Read the model definition and answer for the solid it produces. Units are mm, in the model's axes. A direction names the side the tool comes from. Coordinates: 2 decimals unless noted, no trailing zeros. Order: outer loops, then holes, each group sorted by start corner. A loop starts at its lowest first (then second) coordinate and runs counter-clockwise, first axis right, second up. Notation, with made-up numbers: (34.25, 31) -> (72.25, 31) arc R11 ccw to (72.25, 46) -> close; hole circle Ø8 at (8, 64). An arc over 180 degrees is marked (long way). Answer in a Markdown table with one row per item.
from build123d import *

# Parameters (mm, degrees)
SKETCH_1_R          = 7
EXTRUDE_1_DEPTH     = 2
SKETCH_2_R          = 5
EXTRUDE_2_DEPTH     = 5
SKETCH_3_R          = 2.5
CUT_EXTRUDE_1_DEPTH = 5
FILLET_1_R          = 1


with BuildPart() as part:
    # 草图1 → 凸台-拉伸1 (new body)
    with BuildSketch(Plane(origin=(0, 0, 0), x_dir=(1, 0, 0), z_dir=(0, 1, 0))):
        Circle(SKETCH_1_R)
    extrude(amount=EXTRUDE_1_DEPTH)

    # 草图2 → 凸台-拉伸2 (add)
    with BuildSketch(Plane(origin=(0, 2, 0), x_dir=(1, 0, 0), z_dir=(0, 1, 0))):
        Circle(SKETCH_2_R)
    extrude(amount=EXTRUDE_2_DEPTH)

    # 草图3 → 切除-拉伸1 (cut)
    with BuildSketch(Plane.XZ):
        Circle(SKETCH_3_R)
    extrude(amount=-CUT_EXTRUDE_1_DEPTH, mode=Mode.SUBTRACT)

    # 圆角1
    fillet_1_edges = [part.edges().sort_by_distance(p)[0] for p in [
        (-5, 7, 0),
    ]]
    fillet(fillet_1_edges, radius=FILLET_1_R)


solid = part.part
Q1. For faces 1 (the face through (-1.08, 3.97, 4.88)), 2 (the face through (-0.54, 2.46, -2.44)), 3 (the face through (0, 7, 0)), determine the directions among +Z, -Z, +X, -X, +Y, -Y from which every point of the face is accessible in a straight line to the end or side of a thin tool.
Outcome:
| item | result |
|---|---|
| face 1 | +Y |
| face 2 | -Y |
| face 3 | +Z, -Z, +X, -X, +Y |
Q2. Consider line 1 (Z direction, x = 0, y = 3.8); line 2 (Y direction, x = -4.75, z = 2.25); line 3 (Y direction, x = 1, z = 0.5). Determine where each line is inside the solid, lowest interval first.
Outcome:
| item | result |
|---|---|
| line 1 | -5 to -2.5, 2.5 to 5 |
| line 2 | 0 to 2 |
| line 3 | 5 to 7 |
Q3. The part is cut by section A-A (z = 0). Write down the section's boundary in (x, y), then the cut area to 3 significant figures.
Outcome:
| item | result |
|---|---|
| outline | (-7, 0) -> (-2.5, 0) -> (-2.5, 5) -> (2.5, 5) -> (2.5, 0) -> (7, 0) -> (7, 2) -> (5, 2) -> (5, 6) arc R1 ccw to (4, 7) -> (-4, 7) arc R1 ccw to (-5, 6) -> (-5, 2) -> (-7, 2) -> close |
| area | 52.6 mm² |
Q4. For a pull along X with two mould halves and no side action, classify faces 4 (the face through (0, 5, 0)), 5 (the face through (-2, 2, -5)), 6 (the face through (6.466, 0.986, 2.681)) as pulls with the +X half, pulls with the -X half, needs draft (parallel to the pull), parting line crosses it, or undercut.
Outcome:
| item | result |
|---|---|
| face 4 | undercut |
| face 5 | needs draft |
| face 6 | parting line crosses it |
Q5. The part is cut by section C-C (y = 4.5). Write down the section's boundary in (x, z), then the cut area to 3 significant figures.
Outcome:
| item | result |
|---|---|
| outline | circle Ø10 at (0, 0); hole circle Ø5 at (0, 0) |
| area | 58.9 mm² |
Q6. The part is cut by section D-D (y = 1.75). Write down the section's boundary in (x, z).
Outcome:
| item | result |
|---|---|
| outline | circle Ø14 at (0, 0); hole circle Ø5 at (0, 0) |
Q7. The part is cut by section B-B (x = 0). Write down the section's boundary in (y, z), then the cut area to 3 significant figures.
Outcome:
| item | result |
|---|---|
| outline | (0, -7) -> (2, -7) -> (2, -5) -> (6, -5) arc R1 ccw to (7, -4) -> (7, 4) arc R1 ccw to (6, 5) -> (2, 5) -> (2, 7) -> (0, 7) -> (0, 2.5) -> (5, 2.5) -> (5, -2.5) -> (0, -2.5) -> close |
| area | 52.6 mm² |
Q8. Given pin 1 (2.5 mm diameter, centred on x = 0.5, z = -1, fed in from -Y); pin 2 (1.5 mm diameter, centred on x = -2.5, y = 3, fed in from +Z); pin 3 (3 mm diameter, centred on x = 1.5, y = 5, fed in from +Z); pin 4 (6 mm diameter, centred on x = -1.5, z = 1.5, fed in from -Y), each flat-ended and moving along its own axis, determine where each tip first touches the part or whether it passes through.
Outcome:
| item | result |
|---|---|
| pin 1 | y = 5 |
| pin 2 | z = 4.68 |
| pin 3 | z = 5 |
| pin 4 | y = 0 |
